Source: three-view drawing plus pictorial views. Frame: mm from the lowest corner of the part. A direction names the side the tool comes from. Give positions to 0.01 mm unless a question says otherwise; leave off trailing zeros. Loops run counter-clockwise (first coordinate to the right, second up) from the corner with the lowest first, then second, coordinate; pieces in that order, holes last. Notation, with made-up numbers: (22, 70.25) - (53, 70.25) arc R13 ccw to (53, 89.25) - close; hole circle Ø6 at (70.5, -24). An arc over 180 degrees is marked (long way). Write each question's results on one line, items separated by ' | '. Start each with the question number.
(1) Reachability of the marked faces 4, 5 and 6 from +Z, -Z, +X, -X, +Y, -Y: full face, straight path, thin tool, end or side. Return the list, or none.
(2) Cut plane D-D on z = 92. Return the cut outline in (x, y), then the cut area to 3 significant figures.
(3) Pull-direction query (X, two-part tool) for the marked faces 1, 2 and 3; classes: pulls with the +X half, pulls with the -X half, needs draft (parallel to the pull), parting line crosses it, or undercut.
(4) Material intervals for line 1 along X through (y, z) = (18.75, 29); line 2 along Z through (x, y) = (129, 13.5); line 3 along Z through (x, y) = (97.5, 18.25), sorted ascending. Write a range as [from, to].
(5) Cut plane B-B on x = 29. Return the cut outline in (y, z).
(6) Cut plane C-C on y = 19.5. Return the cut outline in (x, z), then the cut area to 3 significant figures.
(7) Contact query for flat-ended pins moving along their axis: pin 1 (1 mm diameter, centred on y = 9, z = 66, fed in from -X); pin 2 (1 mm diameter, centred on x = 24, y = 13, fed in from -Z); pin 3 (12 mm diameter, centred on y = 11.5, z = 72.5, fed in from +X). Output: stop coordinate, or through.
(8) Cut plane A-A on z = 29. Return the cut outline in (x, y).
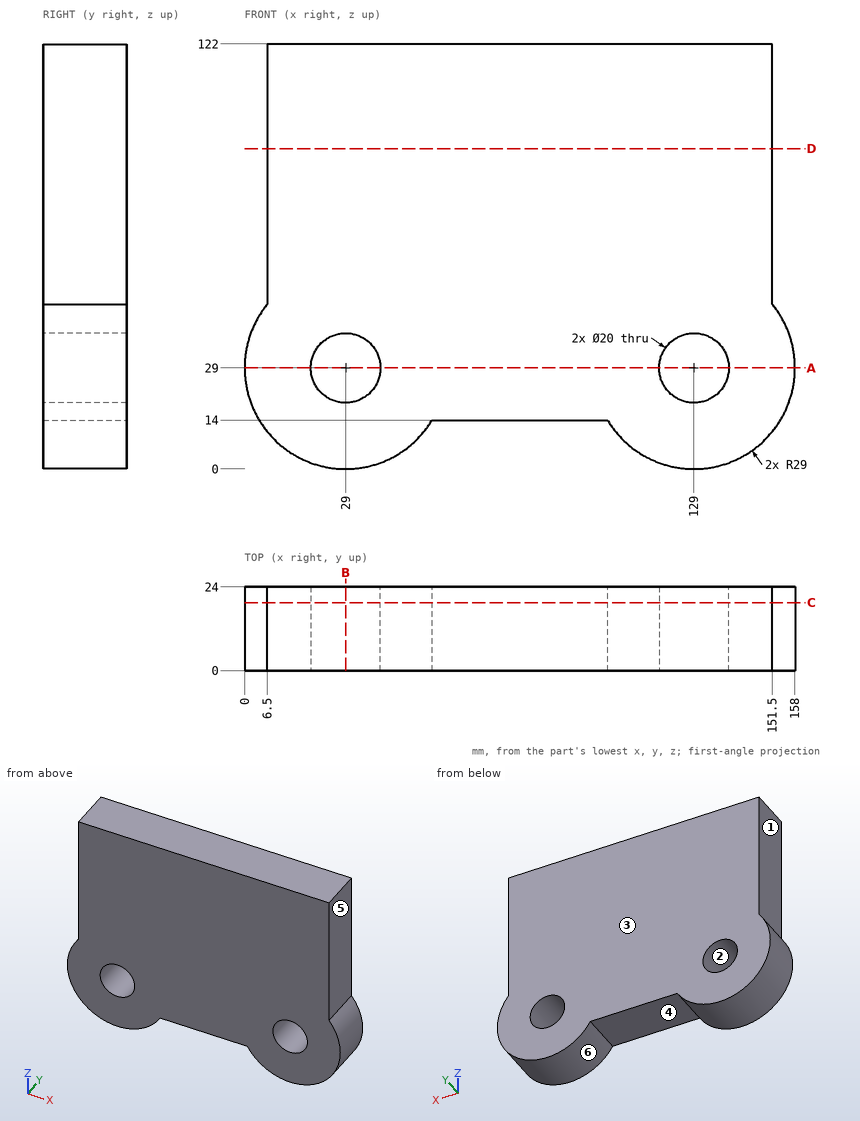
Ans:
1) face 4: -Z, +Y, -Y | face 5: +Z, +X, +Y, -Y | face 6: +Y, -Y
2) outline: (6.5, 0) - (151.5, 0) - (151.5, 24) - (6.5, 24) - close | area: 3,480 mm^2
3) face 1: pulls with the -X half | face 2: undercut | face 3: needs draft
4) line 1: [0, 19], [39, 119], [139, 158] | line 2: [0, 19], [39, 122] | line 3: [14, 122]
5) outline: (0, 0) - (24, 0) - (24, 19) - (0, 19) - close; (0, 39) - (24, 39) - (24, 122) - (0, 122) - close
6) outline: (6.5, 47.3) arc R29 ccw (long way) to (53.82, 14) - (104.18, 14) arc R29 ccw (long way) to (151.5, 47.3) - (151.5, 122) - (6.5, 122) - close; hole circle Ø20 at (29, 29); hole circle Ø20 at (129, 29) | area: 16,300 mm^2
7) pin 1: x = 6.5 | pin 2: z = 0.35 | pin 3: x = 151.5
8) outline: (0, 0) - (19, 0) - (19, 24) - (0, 24) - close; (39, 0) - (119, 0) - (119, 24) - (39, 24) - close; (139, 0) - (158, 0) - (158, 24) - (139, 24) - close
